Input: part model. Units: mm. Frame: model coordinates. A direction names the side the tool comes from. Coordinates: 2 decimals unless noted, no trailing zeros. Loops run counter-clockwise (first coordinate to the right, second up) from the corner with the lowest first, then second, coordinate; pieces in that order, holes last.
(1) Section B-B, the plane x = 0. Return loops of the section in (y, z), then the cut area to 3 significant figures.
(2) Line query: L1, parallel to Z at x = 0, y = -174; L2, parallel to Y at x = -4, z = 8.5; L3, parallel to X at y = -290, z = -0.5. Output: solid intervals per line, ascending.
(3) Mould query, pull axis Y, two halves, no side actions, for faces 1 (the face through (0, 17, 0)), 2 (the face through (0, -317, 0)), 3 (the face through (-2.38, -308.38, 10.74)), 4 (the face through (-2.17, -147.9, -9.76)). Classes: released by +Y, released by -Y, zero draft, split by the parting line, or undercut.
(4) Set-up query: faces 5 (the face through (2, -300, 10)), 6 (the face through (-2.38, 8.38, 10.74)). Return all of +Z, -Z, +X, -X, +Y, -Y with unobstructed straight access to the full face (end or side cutting, diameter ignored); none if empty.
(5) Section C-C, the plane y = -249. Return loops of the section in (x, z), then the cut area to 3 significant figures.
(6) Section A-A, the plane z = 0. Return loops of the section in (x, y), then the cut area to 3 significant figures.
(7) Contact query for flat-ended pins moving along their axis: P1, Ø6, axis at y = -210.5, z = 1.5, coming from the -X side; P2, Ø6, axis at y = -61, z = 7.5, coming from the -X side; P3, Ø5, axis at x = -5.5, y = -283.5, coming from the +Z side. Output: stop coordinate, or through.
```python
from build123d import *

# Parameters (mm, degrees)
F0_R     = 10
F0_R_2   = 9.5
F1_DEPTH = 300


with BuildPart() as f1:
    # F0 (on Front) → F1 (new body)
    with BuildSketch(Plane.XZ):
        Circle(F0_R)
        Circle(F0_R_2, mode=Mode.SUBTRACT)
    extrude(amount=F1_DEPTH)

    # F2 (on Top) → F3 (revolve)
    with BuildSketch(Plane.XY):
        Polygon((11, -300), (0, -300), (0, -317), (1.930615992, -317), (11, -317), align=None)
    revolve(axis=Axis((0, -515.2761181587, 0), (0, 1, 0)))

    # F5: F1 across plane


with BuildPart() as f1_1:
    add(f1.part)
    add(f1.part.mirror(Plane(origin=(0, -150, 0), x_dir=(1, 0, 0), z_dir=(0, 1, 0))))


solid = f1_1.part
```
Report:
1. outline: (-317, -11) - (-300, -11) - (-300, -10) - (0, -10) - (0, -11) - (17, -11) - (17, 11) - (0, 11) - (0, 10) - (-300, 10) - (-300, 11) - (-317, 11) - close; hole (-300, -9.5) - (0, -9.5) - (0, 9.5) - (-300, 9.5) - close
1. area: 1,050 mm2
2. L1: z = -10 to -9.5, 9.5 to 10
2. L2: y = -317 to -300, 0 to 17
2. L3: x = -9.99 to -9.49, 9.49 to 9.99
3. face 1: released by +Y
3. face 2: released by -Y
3. face 3: zero draft
3. face 4: undercut
4. face 5: none
4. face 6: +Y, -Y
5. outline: circle Ø20 at (0, 0); hole circle Ø19 at (0, 0)
5. area: 30.6 mm2
6. outline: (-11, -317) - (11, -317) - (11, -300) - (10, -300) - (10, 0) - (11, 0) - (11, 17) - (-11, 17) - (-11, 0) - (-10, 0) - (-10, -300) - (-11, -300) - close; hole (-9.5, -300) - (9.5, -300) - (9.5, 0) - (-9.5, 0) - close
6. area: 1,050 mm2
7. P1: stops at x = -10
7. P2: stops at x = -8.93
7. P3: stops at z = 9.54
